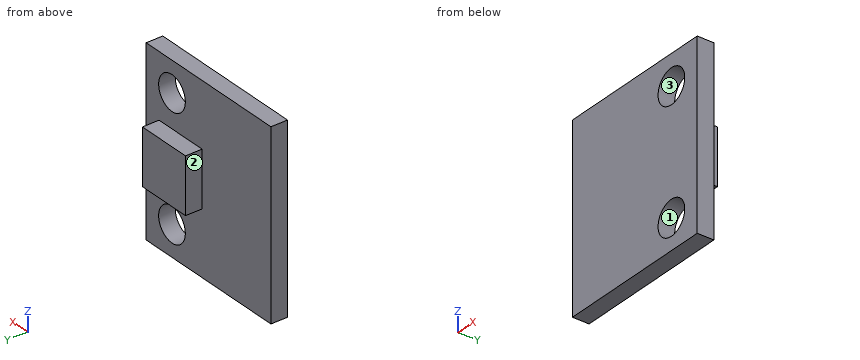
from build123d import *

# Parameters (mm, degrees)
SKETCH1_W           = 14.5
SKETCH1_H           = 16.5
BOSS_EXTRUDE1_DEPTH = 1.5
SKETCH2_R           = 1.55
CUT_EXTRUDE1_DEPTH  = 12.084899639
SKETCH3_W           = 5
SKETCH3_H           = 5
BOSS_EXTRUDE2_DEPTH = 1.5


with BuildPart() as part:
    # Sketch1 → Boss-Extrude1 (new body)
    with BuildSketch(Plane(origin=(0, 0, 0), x_dir=(1, 0, 0), z_dir=(0, 1, 0))):
        Rectangle(SKETCH1_W, SKETCH1_H)
    extrude(amount=BOSS_EXTRUDE1_DEPTH)

    # Sketch2 → Cut-Extrude1 (cut, through all)
    with BuildSketch(Plane(origin=(0, 1.5, 0), x_dir=(1, 0, 0), z_dir=(0, 1, 0))):
        with Locations(Location((4.25, 5.5, 0), (0, 0, 270))):
            Circle(SKETCH2_R)
        with Locations(Location((4.25, -5.5, 0), (0, 0, 90))):
            Circle(SKETCH2_R)
    extrude(amount=-CUT_EXTRUDE1_DEPTH, mode=Mode.SUBTRACT)

    # Sketch3 → Boss-Extrude2 (add)
    with BuildSketch(Plane(origin=(0, 1.5, 0), x_dir=(1, 0, 0), z_dir=(0, 1, 0))):
        with Locations((3.25, 0)):
            Rectangle(SKETCH3_W, SKETCH3_H)
    extrude(amount=BOSS_EXTRUDE2_DEPTH)


solid = part.part
Here's how the part is built. I have some questions about the finished solid (model axes, mm). Face numbers are marked on the shaded views. Coordinates: 2 decimals unless noted, no trailing zeros. Loops run counter-clockwise (first coordinate to the right, second up) from the corner with the lowest first, then second, coordinate; pieces in that order, holes last.
1. Imagine slicing it at D-D, the plane x = 1.5. Please give me the cut outline in (y, z).
2. Imagine slicing it at C-C, the plane y = 1.3. Please give me the cut outline in (x, z).
3. I need wall thicknesses on L1, parallel to X at y = 1.1, z = -5.5; L2, parallel to Z at x = 4, y = 1.35; L3, parallel to Y at x = 4, z = 3.25. Which ranges of each line are inside material? Lowest first, please.
4. If we mould it in two halves opening along Z, with no side actions, what happens to the marked faces 1, 2 and 3? For each: pulls with the +Z half, pulls with the -Z half, needs draft (parallel to the pull), parting line crosses it, or undercut.
5. Imagine slicing it at B-B, the plane x = 4.25. Please give me the cut outline in (y, z).
6. For P1, Ø1.2, axis at x = 2.5, y = 2.5, coming from the -Z side; P2, Ø0.8, axis at x = 3, y = 2, coming from the +Z side; P3, Ø3.5, axis at x = 4.25, z = -5.5, coming from the +Y side, each with a flat end and sliding along its axis, tell me the tip position at first contact or that it passes through.
7. Imagine slicing it at A-A, the plane z = 5.5. Please give me the cut outline in (x, y), and give its area (3 significant figures).
Taken from the geometry:
1. outline: (0, -8.25) - (1.5, -8.25) - (1.5, -2.5) - (3, -2.5) - (3, 2.5) - (1.5, 2.5) - (1.5, 8.25) - (0, 8.25) - close
2. outline: (-7.25, -8.25) - (7.25, -8.25) - (7.25, 8.25) - (-7.25, 8.25) - close; hole circle Ø3.1 at (4.25, -5.5); hole circle Ø3.1 at (4.25, 5.5)
3. L1: x = -7.25 to 2.7, 5.8 to 7.25
3. L2: z = -8.25 to -7.03, -3.97 to 3.97, 7.03 to 8.25
3. L3: y = 0 to 1.5
4. face 1: undercut
4. face 2: needs draft
4. face 3: undercut
5. outline: (0, -8.25) - (1.5, -8.25) - (1.5, -7.05) - (0, -7.05) - close; (0, -3.95) - (1.5, -3.95) - (1.5, -2.5) - (3, -2.5) - (3, 2.5) - (1.5, 2.5) - (1.5, 3.95) - (0, 3.95) - close; (0, 7.05) - (1.5, 7.05) - (1.5, 8.25) - (0, 8.25) - close
6. P1: stops at z = -2.5
6. P2: stops at z = 2.5
6. P3: stops at y = 1.5
7. outline: (-7.25, 0) - (2.7, 0) - (2.7, 1.5) - (-7.25, 1.5) - close; (5.8, 0) - (7.25, 0) - (7.25, 1.5) - (5.8, 1.5) - close
7. area: 17.1 mm2
